For this review, take the finished solid that the model builds, in its own axes (mm). A direction names the side the tool comes from. Give positions to 0.01 mm unless a question says otherwise; leave off trailing zeros. Write each loop counter-clockwise with the first axis right and the second up, starting at its lowest first coordinate (ties: lowest second). Pieces come first, ordered by that corner, then holes.
1) Wall thickness on line 1 along Y through (x, z) = (280, 13.85); line 2 along Y through (x, z) = (-5, 12.05); line 3 along Y through (x, z) = (-5, 14.35): over which ranges is each line inside the solid? List them lowest first.
2) For P1, Ø3.5, axis at x = 204, y = -12.5, coming from the +Z side; P2, Ø2, axis at x = 150, z = 11.5, coming from the +Y side; P3, Ø3, axis at x = -3.5, z = 13, coming from the -Y side, all flat-tipped, find the tip position at first contact; note any pin that passes through.
3) We need section A-A on z = 11.1. Give the number of separate pieces and of enclosed holes in the cut face, and give its area (3 significant figures).
4) We need section C-C on x = 227. Give the boundary of the cut face in (y, z), and give its area (3 significant figures).
5) Machinability: for faces 1 (the face through (-18.9, 24.8, 13.5)), 2 (the face through (172.244, -5.485, 12.465)), 3 (the face through (-31.21, 34.53, 13.82)), 4 (the face through (-34.72, -20.02, 12.46)), 5 (the face through (128, 34, 10)), which of the approach directions +Z, -Z, +X, -X, +Y, -Y give a long, thin tool a straight path to every point of the face, cutting with its end or side? Answer none if there is none.
6) We need section B-B on x = 27. Give the boundary of the cut face in (y, z).
from build123d import *

# Parameters (mm, degrees)
DODANIE_WYCI_GNI_CIE1_DEPTH = 5
SZKIC1_R                    = 3.5
WYTNIJ_WYCI_GNI_CIE1_DEPTH  = 100
SZKIC3_R                    = 1.5
WYTNIJ_WYCI_GNI_CIE3_DEPTH  = 5
SZKIC5_R                    = 3
WYTNIJ_WYCI_GNI_CIE4_DEPTH  = 2.4


with BuildPart() as part:
    # outer-wire → Dodanie-wyciągnięcie1 (new body)
    with BuildSketch(Plane.XY):
        with BuildLine():
            Line((-24, -24.53020641), (62.5, -24.53020641))
            ThreePointArc((62.5, -24.53020641), (65.803504247, -23.968789974), (68.736080178, -22.347578348))
            Line((68.736080178, -22.347578348), (89, -6.182628062))
            ThreePointArc((89, -6.182628062), (91.932575931, -4.561416436), (95.236080178, -4))
            Line((95.236080178, -4), (167, -4))
            ThreePointArc((167, -4), (172.310885546, -5.526836794), (176, -9.641101056))
            Line((176, -9.641101056), (192, -39.280484771))
            ThreePointArc((192, -39.280484771), (195.676368139, -43.118069462), (200.799707694, -44.53020641))
            Line((200.799707694, -44.53020641), (271, -44.53020641))
            ThreePointArc((271, -44.53020641), (292.697243682, -34.454979346), (299, -11.3778078))
            Line((299, -11.3778078), (299, 70.236479581))
            ThreePointArc((299, 70.236479581), (290.082226047, 86.530998263), (273, 93.827270232))
            Line((273, 93.827270232), (-19, 110))
            ThreePointArc((-19, 110), (-33.142135624, 104.142135624), (-39, 90))
            Line((-39, 90), (-39, -9.53020641))
            ThreePointArc((-39, -9.53020641), (-34.606601718, -20.136808128), (-24, -24.53020641))
        make_face()
    extrude(amount=DODANIE_WYCI_GNI_CIE1_DEPTH)

    # Szkic1 → Wytnij-wyciągnięcie1 (cut)
    with BuildSketch(Plane(origin=(0, -24.53020641, 0), x_dir=(-1, 0, 0), z_dir=(0, -1, 0))):
        with Locations((19, 0)):
            Circle(SZKIC1_R)
    extrude(amount=-WYTNIJ_WYCI_GNI_CIE1_DEPTH, mode=Mode.SUBTRACT)

    # Szkic3 → Wytnij-wyciągnięcie3 (cut)
    with BuildSketch(Plane.XY.offset(5)):
        with Locations((280, -28)):
            Circle(SZKIC3_R)
        with Locations((280, 77.5)):
            Circle(SZKIC3_R)
        with Locations((-5, 77.5)):
            Circle(SZKIC3_R)
        with Locations((-29, 77.5)):
            Circle(SZKIC3_R)
        with Locations((-29, -12.5)):
            Circle(SZKIC3_R)
        with Locations((-29, 32.5)):
            Circle(SZKIC3_R)
        with Locations((-5, 32.5)):
            Circle(SZKIC3_R)
        with Locations((-5, -12.5)):
            Circle(SZKIC3_R)
        with Locations((60, -12.5)):
            Circle(SZKIC3_R)
        with Locations((204, -12.5)):
            Circle(SZKIC3_R)
        with Locations((137.5, 77.5)):
            Circle(SZKIC3_R)
    extrude(amount=-WYTNIJ_WYCI_GNI_CIE3_DEPTH, mode=Mode.SUBTRACT)

    # Szkic5 → Wytnij-wyciągnięcie4 (cut)
    with BuildSketch(Plane.XY.offset(5)):
        with Locations((-29, -12.5)):
            Circle(SZKIC5_R)
        with Locations((-29, 32.5)):
            Circle(SZKIC5_R)
        with Locations((-29, 77.5)):
            Circle(SZKIC5_R)
        with Locations((-5, 77.5)):
            Circle(SZKIC5_R)
        with Locations((-5, 32.5)):
            Circle(SZKIC5_R)
        with Locations((-5, -12.5)):
            Circle(SZKIC5_R)
        with Locations((60, -12.5)):
            Circle(SZKIC5_R)
        with Locations((137.5, 77.5)):
            Circle(SZKIC5_R)
        with Locations((204, -12.5)):
            Circle(SZKIC5_R)
        with Locations((280, -28)):
            Circle(SZKIC5_R)
        with Locations((280, 77.5)):
            Circle(SZKIC5_R)
    extrude(amount=-WYTNIJ_WYCI_GNI_CIE4_DEPTH, mode=Mode.SUBTRACT)


with BuildPart() as body_2:
    # Lustro4: mirrored copy
    add(part.part.mirror(Plane.XY.offset(5)))


with BuildPart() as body_2_2:
    # Lustro5: mirrored copy
    add(body_2.part.mirror(Plane(origin=(-24, -9.53020641, 10), x_dir=(1, 0, 0), z_dir=(0, 0, -1))))


with BuildPart() as body_2_3:
    # Lustro6: mirrored copy
    add(body_2_2.part.mirror(Plane(origin=(-24, -9.53020641, 10), x_dir=(1, 0, 0), z_dir=(0, 0, 1))))


with BuildPart() as body_2_4:
    # Lustro7: mirrored copy
    add(body_2_3.part.mirror(Plane(origin=(-24, -9.53020641, 10), x_dir=(1, 0, 0), z_dir=(0, 0, -1))))


solid = body_2_4.part
Results list:
1. line 1: y = -43.07 to -31, -25 to 74.5, 80.5 to 92.43
1. line 2: y = -24.53 to -14, -11 to 31, 34 to 76, 79 to 109.22
1. line 3: y = -24.53 to -15.5, -9.5 to 29.5, 35.5 to 74.5, 80.5 to 109.22
2. P1: stops at z = 12.6
2. P2: stops at y = 100.7
2. P3: stops at y = -24.53
3. separate pieces: 1
3. enclosed holes: 11
3. area: 41,600 mm2
4. outline: (-44.53, 10) - (96.38, 10) - (96.38, 15) - (-44.53, 15) - close
4. area: 705 mm2
5. face 1: -Z, -Y
5. face 2: +Z, -Z, -Y
5. face 3: +Z
5. face 4: +Z, -Z, -X, -Y
5. face 5: -Z, +X, -X, +Y, -Y
6. outline: (-24.53, 10) - (107.45, 10) - (107.45, 15) - (-24.53, 15) - close
